Can you work these out from the model? Positions are in its coordinate system, mm. Face numbers are marked on the shaded views. Round coordinates to 2 decimals unless told otherwise and drop trailing zeros. Loops run counter-clockwise (first coordinate to the right, second up) from the corner with the lowest first, then second, coordinate; pieces in that order, holes last. Notation, with made-up numbers: (21.5, -14) -> (71.5, -14) arc R20 cw to (71.5, 20) -> close; hole circle Ø11 at (48, -4.75). An arc over 180 degrees is marked (long way). Answer as a JSON object with one key per item and string values.
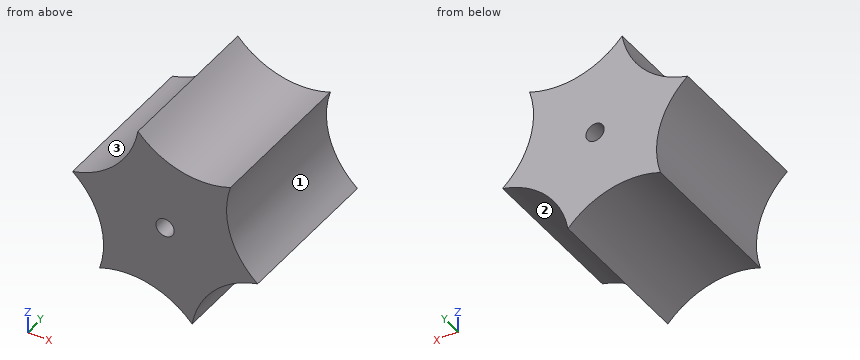
```python
from build123d import *

# Parameters (mm, degrees)
F0_R     = 0.75
F1_DEPTH = 13


with BuildPart() as f1:
    # F0 (on Front) → F1 (new body)
    with BuildSketch(Plane.XZ):
        with BuildLine():
            ThreePointArc((-45.877073, 37.077873), (-47.700367, 33.412388), (-51.261876, 31.393517))
            ThreePointArc((-51.261876, 31.393517), (-48.99912, 27.981756), (-49.031481, 23.887964))
            ThreePointArc((-49.031481, 23.887964), (-44.945431, 24.141687), (-41.416284, 22.066766))
            ThreePointArc((-41.416284, 22.066766), (-39.592989, 25.732251), (-36.031481, 27.751121))
            ThreePointArc((-36.031481, 27.751121), (-38.294237, 31.162883), (-38.261876, 35.256675))
            ThreePointArc((-38.261876, 35.256675), (-42.347926, 35.002951), (-45.877073, 37.077873))
        make_face()
        with Locations((-43.646678, 29.572319)):
            Circle(F0_R, mode=Mode.SUBTRACT)
    extrude(amount=F1_DEPTH)


solid = f1.part
```
Q1. I want a section at C-C, the plane x = -39.75. Write out the boundary of the cut face in (y, z), then the cut area to 3 significant figures.
Determined:
{"outline": "(-13, 25.56) -> (0, 25.56) -> (0, 34.88) -> (-13, 34.88) -> close", "area": "121 mm²"}
Q2. We'd pull the mould along Z, two halves only. Please class the marked faces 1, 2 and 3: pulls with the +Z half, pulls with the -Z half, needs draft (parallel to the pull), parting line crosses it, or undercut.
Determined:
{"face 1": "undercut", "face 2": "pulls with the -Z half", "face 3": "pulls with the +Z half"}
Q3. I want a section at B-B, the plane z = 27. Write out the boundary of the cut face in (x, y), then the cut area to 3 significant figures.
Determined:
{"outline": "(-48.78, -13) -> (-37.98, -13) -> (-37.98, 0) -> (-48.78, 0) -> close", "area": "140 mm²"}
Q4. I want a section at A-A, the plane y = -3.25. Write out the boundary of the cut face in (x, z), then the cut area to 3 significant figures.
Determined:
{"outline": "(-51.26, 31.39) arc R7 cw to (-49.03, 23.89) arc R7 cw to (-41.42, 22.07) arc R7 cw to (-36.03, 27.75) arc R7 cw to (-38.26, 35.26) arc R7 cw to (-45.88, 37.08) arc R7 cw to start; hole circle Ø1.5 at (-43.65, 29.57)", "area": "119 mm²"}
Q5. I'm going to push flat-ended pins straight in: pin 1 (4 mm diameter, centred on x = -37.5, y = -5.5, fed in from -Z); pin 2 (4 mm diameter, centred on y = -3, z = 35.5, fed in from -X); pin 3 (1.5 mm diameter, centred on y = -4.5, z = 29.5, fed in from -X); pin 4 (5 mm diameter, centred on x = -42.5, z = 30, fed in from +Y). Where does each tip first touch, or does it pass through?
Determined:
{"pin 1": "z = 25.83", "pin 2": "x = -47.62", "pin 3": "x = -50.16", "pin 4": "y = 0"}
Q6. If I drill on L1, parallel to X at y = -4.75, z = 30.25; L2, parallel to Z at x = -50.5, y = -2.25; L3, parallel to X at y = -3.5, z = 30.75, over which ranges is the centre line in solid material (lowest first)? Write a range as [from, to].
Determined:
{"L1": "[-50.16, -43.97], [-43.33, -37.95]", "L2": "[30.66, 31.61]", "L3": "[-50.58, -38.16]"}
